Geometry: final body of the model. Coordinates: model frame, mm. Face numbers are marked on the shaded views. A direction names the side the tool comes from. Round coordinates to 2 decimals unless told otherwise and drop trailing zeros. Loops run counter-clockwise (first coordinate to the right, second up) from the corner with the lowest first, then second, coordinate; pieces in that order, holes last. Notation, with made-up numbers: (26, 58) -> (59, 58) arc R16 ccw to (59, 64) -> close; hole circle Ø7 at (70, 77). An arc over 180 degrees is marked (long way). Answer in a Markdown table with one row per item.
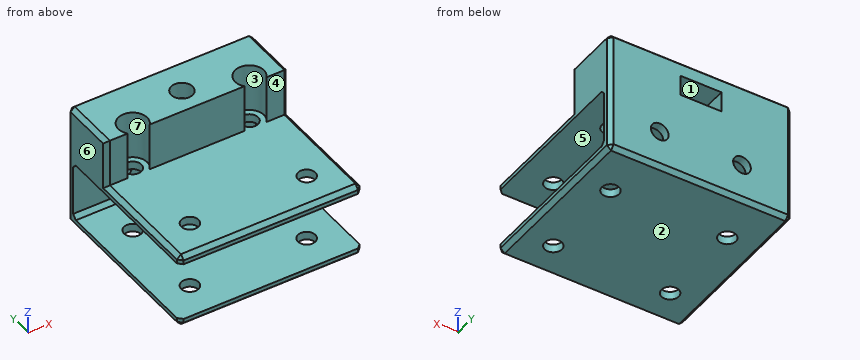
```python
from build123d import *

# Parameters (mm, degrees)
SKETCH1_W           = 44.4
SKETCH1_H           = 40
SKETCH1_R           = 2.1
BOSS_EXTRUDE1_DEPTH = 2
SKETCH2_W           = 44.4
SKETCH2_H           = 18.3
BOSS_EXTRUDE2_DEPTH = 2
LPATTERN1_COUNT     = 2
LPATTERN1_PITCH     = 16.3
SKETCH3_R           = 2.15
CUT_EXTRUDE1_DEPTH  = 64.253853638
BOSS_EXTRUDE3_START = -22.2
SKETCH6_W           = 11.69
SKETCH6_H           = 14.27
BOSS_EXTRUDE3_DEPTH = 44.4
CUT_EXTRUDE2_REACH  = 70.079
SKETCH7_R           = 2.6
CUT_EXTRUDE3_REACH  = 65.254
SKETCH8_R           = 2.1
SKETCH9_R           = 3.5
CUT_EXTRUDE4_DEPTH  = 11.69
FILLET4_SIZE        = 1
SKETCH11_W          = 10
SKETCH11_H          = 5
CUT_EXTRUDE6_DEPTH  = 12.27


with BuildPart() as part:
    # Sketch1 → Boss-Extrude1 (new body)
    with BuildSketch(Plane.XY):
        with Locations((22.2, 20)):
            Rectangle(SKETCH1_W, SKETCH1_H)
        with Locations((8, 8.476902454)):
            Circle(SKETCH1_R, mode=Mode.SUBTRACT)
        with Locations((8, 29.976902454)):
            Circle(SKETCH1_R, mode=Mode.SUBTRACT)
        with Locations((36.4, 29.976902454)):
            Circle(SKETCH1_R, mode=Mode.SUBTRACT)
        with Locations((36.4, 8.476902454)):
            Circle(SKETCH1_R, mode=Mode.SUBTRACT)
    boss_extrude1 = extrude(amount=BOSS_EXTRUDE1_DEPTH)

    # Sketch2 → Boss-Extrude2 (add)
    with BuildSketch(Plane(origin=(0, 40, 0), x_dir=(1, 0, 0), z_dir=(0, 1, 0))):
        with Locations((22.2, 7.15)):
            Rectangle(SKETCH2_W, SKETCH2_H)
    extrude(amount=BOSS_EXTRUDE2_DEPTH)

    # LPattern1: Boss-Extrude1 ×2
    with Locations(*[(0, 0, -i * LPATTERN1_PITCH) for i in range(1, LPATTERN1_COUNT)]):
        add(boss_extrude1)

    # Sketch3 → Cut-Extrude1 (cut, through all)
    with BuildSketch(Plane(origin=(0, 42, 0), x_dir=(1, 0, 0), z_dir=(0, 1, 0))):
        with Locations(Location((12.2, 7.15, 0), (0, 0, 270))):
            Circle(SKETCH3_R)
        with Locations(Location((32.2, 7.15, 0), (0, 0, 270))):
            Circle(SKETCH3_R)
    extrude(amount=-CUT_EXTRUDE1_DEPTH, mode=Mode.SUBTRACT)

    # Sketch6 → Boss-Extrude3 (add)
    with BuildSketch(Plane(origin=(22.2, 0, 0), x_dir=(0, 0, -1), z_dir=(1, 0, 0)).offset(BOSS_EXTRUDE3_START)):
        with Locations((-7.845, 34.865)):
            Rectangle(SKETCH6_W, SKETCH6_H)
    extrude(amount=BOSS_EXTRUDE3_DEPTH)

    # Sketch7 → Cut-Extrude2 (cut, up to next)
    with BuildSketch(Plane.XY.offset(13.69), mode=Mode.PRIVATE) as cut_extrude2_sk1:
        with Locations((22.2, 33.43)):
            Circle(SKETCH7_R)
    cut_extrude2_tool1 = extrude(cut_extrude2_sk1.sketch, amount=-CUT_EXTRUDE2_REACH, mode=Mode.PRIVATE) & part.part
    add(cut_extrude2_tool1.solids().sort_by_distance((22.2, 33.43, 13.69))[0], mode=Mode.SUBTRACT)

    # Sketch8 → Cut-Extrude3 (cut, up to next)
    with BuildSketch(Plane(origin=(0, 0, 0), x_dir=(-1, 0, 0), z_dir=(0, 0, -1)), mode=Mode.PRIVATE) as cut_extrude3_sk1:
        with Locations(Location((-36.4, 29.976902454, 0), (0, 0, 90))):
            Circle(SKETCH8_R)
    cut_extrude3_tool1 = extrude(cut_extrude3_sk1.sketch, amount=-CUT_EXTRUDE3_REACH, mode=Mode.PRIVATE) & part.part
    # Sketch8 → Cut-Extrude3 (cut, up to next)
    with BuildSketch(Plane(origin=(0, 0, 0), x_dir=(-1, 0, 0), z_dir=(0, 0, -1)), mode=Mode.PRIVATE) as cut_extrude3_sk2:
        with Locations(Location((-8, 29.976902454, 0), (0, 0, 90))):
            Circle(SKETCH8_R)
    cut_extrude3_tool2 = extrude(cut_extrude3_sk2.sketch, amount=-CUT_EXTRUDE3_REACH, mode=Mode.PRIVATE) & part.part
    add(cut_extrude3_tool1.solids().sort_by_distance((36.4, 29.976902, 0))[0], mode=Mode.SUBTRACT)
    add(cut_extrude3_tool2.solids().sort_by_distance((8, 29.976902, 0))[0], mode=Mode.SUBTRACT)

    # Sketch9 → Cut-Extrude4 (cut)
    with BuildSketch(Plane.XY.offset(13.69)):
        with Locations((8, 29.976902454)):
            Circle(SKETCH9_R)
        with Locations((36.4, 29.976902454)):
            Circle(SKETCH9_R)
    extrude(amount=-CUT_EXTRUDE4_DEPTH, mode=Mode.SUBTRACT)

    # Fillet4
    fillet4_edges = [part.edges().sort_by_distance(p)[0] for p in [
        (44.4, 13.865, 2),
        (0, 21, -16.3),
        (44.4, 21, -16.3),
        (0, 42, -1.305),
        (44.4, 42, -1.305),
        (22.2, 42, -16.3),
        (22.2, 40, -14.3),
        (22.2, 0, -16.3),
        (0, 0, -15.3),
        (44.4, 0, -15.3),
        (22.2, 40, 0),
        (0, 13.865, 2),
        (44.4, 27.73, 7.845),
        (44.4, 34.865, 13.69),
        (22.2, 42, 13.69),
        (0, 27.73, 7.845),
        (0, 34.865, 13.69),
        (44.4, 0, 1),
        (0, 0, 1),
        (22.2, 0, 2),
    ]]
    chamfer(fillet4_edges, length=FILLET4_SIZE)

    # Sketch11 → Cut-Extrude6 (cut)
    with BuildSketch(Plane(origin=(0, 42, 0), x_dir=(1, 0, 0), z_dir=(0, 1, 0))):
        with Locations((22.2, -7.19)):
            Rectangle(SKETCH11_W, SKETCH11_H)
    extrude(amount=-CUT_EXTRUDE6_DEPTH, mode=Mode.SUBTRACT)


solid = part.part
```
Item 1: Cut plane D-D (z = -7.15). Output: boundary loops of the cut face in (x, y), then the cut area to 3 significant figures.
Answer:
| item | result |
|---|---|
| outline | (0, 40) -> (10.05, 40) -> (10.05, 42) -> (1, 42) -> (0, 41) -> close; (14.35, 40) -> (30.05, 40) -> (30.05, 42) -> (14.35, 42) -> close; (34.35, 40) -> (44.4, 40) -> (44.4, 41) -> (43.4, 42) -> (34.35, 42) -> close |
| area | 70.6 mm² |
Item 2: Line query: probe 1 along X at (y, z) = (40.4, -7.15); probe 2 along Z at (x, y) = (23.5, 15); probe 3 along X at (y, z) = (41.65, -7.15). Output: solid intervals per line, ascending. Write a range as [from, to].
Answer:
| item | result |
|---|---|
| probe 1 | x = [0, 10.05], [14.35, 30.05], [34.35, 44.4] |
| probe 2 | z = [-16.3, -14.3], [0, 2] |
| probe 3 | x = [0.65, 10.05], [14.35, 30.05], [34.35, 43.75] |
Item 3: Cut plane C-C (x = 32.2). Output: boundary loops of the cut face in (y, z), then the cut area to 3 significant figures.
Answer:
| item | result |
|---|---|
| outline | (0, -15.3) -> (1, -16.3) -> (41, -16.3) -> (42, -15.3) -> (42, -9.3) -> (40, -9.3) -> (40, -13.3) -> (39, -14.3) -> (0, -14.3) -> close; (0, 0) -> (39, 0) -> (40, -1) -> (40, -5) -> (42, -5) -> (42, 12.69) -> (41, 13.69) -> (27.73, 13.69) -> (27.73, 2) -> (1, 2) -> (0, 1) -> close |
| area | 354 mm² |
Item 4: Draft query along Z for the marked faces 1, 2 and 3. Return one class per face: pulls with the +Z half, pulls with the -Z half, needs draft (parallel to the pull), parting line crosses it, or undercut.
Answer:
| item | result |
|---|---|
| face 1 | undercut |
| face 2 | pulls with the -Z half |
| face 3 | needs draft |
Item 5: Reachability of the marked faces 4, 5, 6 and 7 from +Z, -Z, +X, -X, +Y, -Y: full face, straight path, thin tool, end or side. Return the list, or none.
Answer:
| item | result |
|---|---|
| face 4 | +Z, +X, -X, -Y |
| face 5 | +X, -X, -Y |
| face 6 | +Z, -Z, -X, +Y, -Y |
| face 7 | +Z |
Item 6: Cut plane A-A (y = 11.5). Output: boundary loops of the cut face in (x, z).
Answer:
| item | result |
|---|---|
| outline | (0, -15.3) -> (1, -16.3) -> (43.4, -16.3) -> (44.4, -15.3) -> (44.4, -14.3) -> (0, -14.3) -> close; (0, 0) -> (44.4, 0) -> (44.4, 1) -> (43.4, 2) -> (1, 2) -> (0, 1) -> close |
Item 7: Pin query (flat end, axial travel): pin 1 Ø8 at (x, z) = (12, -6.5) entering from -Y; pin 2 Ø1.5 at (x, z) = (17.5, 2.5) entering from -Y; pin 3 Ø4.5 at (x, z) = (40.5, 6) entering from -Y. Return the tip coordinate at first contact, or that it passes through.
Answer:
| item | result |
|---|---|
| pin 1 | stops at y = 40 |
| pin 2 | stops at y = 0.75 |
| pin 3 | stops at y = 27.73 |
Item 8: Cut plane B-B (x = 22.2). Output: boundary loops of the cut face in (y, z), then the cut area to 3 significant figures.
Answer:
| item | result |
|---|---|
| outline | (0, -15.3) -> (1, -16.3) -> (41, -16.3) -> (42, -15.3) -> (42, 4.69) -> (36.03, 4.69) -> (36.03, 0) -> (39, 0) -> (40, -1) -> (40, -13.3) -> (39, -14.3) -> (0, -14.3) -> close; (0, 0) -> (30.83, 0) -> (30.83, 4.69) -> (29.73, 4.69) -> (29.73, 9.69) -> (30.83, 9.69) -> (30.83, 13.69) -> (27.73, 13.69) -> (27.73, 2) -> (1, 2) -> (0, 1) -> close; (36.03, 9.69) -> (42, 9.69) -> (42, 12.69) -> (41, 13.69) -> (36.03, 13.69) -> close |
| area | 256 mm² |
